```python
from build123d import *

# Parameters (mm, degrees)
F0_W     = 90
F0_H     = 55
F1_DEPTH = 35
F2_DEPTH = 7
F3_R     = 10
F4_DEPTH = 5
F6_DEPTH = 90
F7_R     = 4.99999
F8_W     = 12
F8_H     = 3
F9_DEPTH = 30.7
F10_R    = 1


# Not quite as in the source:
# - a fillet or chamfer is up to 0.001 mm smaller than in the source, because OpenCascade refuses the exact size
# - a feature names something its author has since deleted; it is built from what else it names


with BuildPart() as f1:
    # F0 (on Top) → F1 (new body)
    with BuildSketch(Plane.XY):
        Rectangle(F0_W, F0_H)
        with BuildLine():
            ThreePointArc((-40, 0), (-36.0621543344, 11.8032751438), (-25, 17.5))
            ThreePointArc((-25, 17.5), (-13.9378456656, 11.8032751438), (-10, 0))
            ThreePointArc((-10, 0), (-13.9378456656, -11.8032751438), (-25, -17.5))
            ThreePointArc((-25, -17.5), (-36.0621543344, -11.8032751438), (-40, 0))
        make_face(mode=Mode.SUBTRACT)
        with BuildLine():
            ThreePointArc((10, 0), (13.9500894873, 11.8143319509), (25.0340790777, 17.5))
            ThreePointArc((25.0340790777, 17.5), (36.0744106495, 11.7922476991), (40, 0))
            ThreePointArc((40, 0), (36.2593265414, -11.6306402206), (25.5441482581, -17.5))
            ThreePointArc((25.5441482581, -17.5), (14.1318309156, -11.9833988689), (10, 0))
        make_face(mode=Mode.SUBTRACT)
    extrude(amount=F1_DEPTH)

    # F0 (on Top) → F2 (join)
    with BuildSketch(Plane.XY):
        with BuildLine():
            ThreePointArc((-10, 0), (-13.9378456656, 11.8032751438), (-25, 17.5))
            ThreePointArc((-25, 17.5), (-36.0621543344, 11.8032751438), (-40, 0))
            ThreePointArc((-40, 0), (-36.0621543344, -11.8032751438), (-25, -17.5))
            ThreePointArc((-25, -17.5), (-13.9378456656, -11.8032751438), (-10, 0))
        make_face()
        with BuildLine():
            ThreePointArc((40, 0), (36.0744106495, 11.7922476991), (25.0340790777, 17.5))
            ThreePointArc((25.0340790777, 17.5), (13.9500894873, 11.8143319509), (10, 0))
            ThreePointArc((10, 0), (14.1318309156, -11.9833988689), (25.5441482581, -17.5))
            ThreePointArc((25.5441482581, -17.5), (36.2593265414, -11.6306402206), (40, 0))
        make_face()
    extrude(amount=F2_DEPTH)

    # F3 (on face) → F4 (cut)
    with BuildSketch(Plane.XY.offset(7)):
        with Locations((-25, 0)):
            Circle(F3_R)
        with Locations((25.2891136679, 0)):
            Circle(F3_R)
    extrude(amount=-F4_DEPTH, mode=Mode.SUBTRACT)

    # F5 (on face) → F6 (cut)
    with BuildSketch(Plane.YZ.offset(45)):
        Polygon((-27.5, 15), (27.5, 35), (-27.5, 35), align=None)
    extrude(amount=-F6_DEPTH, mode=Mode.SUBTRACT)

    # F7 (radius 5 in the source; OpenCascade refuses exactly that, so slightly less here)
    f7_edges = [f1.edges().sort_by_distance(p)[0] for p in [
        (0, 27.5, 35),
        (-45, 0, 25),
        (0, -27.5, 15),
        (45, 0, 25),
    ]]
    fillet(f7_edges, radius=F7_R)

    # F8 (on face) → F9 (cut)
    with BuildSketch(Plane.XY.offset(7)):
        with Locations((-24.9983986142, 16.138614808)):
            Rectangle(F8_W, F8_H)
        Polygon((32.0340790777, 17.5), (25.0340790777, 17.5), (18.0340790777, 17.5), (18.0340790777, 14.5), (32.0340790777, 14.5), align=None)
    extrude(amount=F9_DEPTH, mode=Mode.SUBTRACT)

    # F10
    f10_edges = [f1.edges().sort_by_distance(p)[0] for p in [
        (-24.998399, 17.638615, 31.414042),
        (-30.998399, 16.709549, 31.0762),
        (-18.998399, 16.708736, 31.075904),
        (32.034079, 16.355367, 30.947406),
        (25.034079, 17.5, 31.363636),
        (18.034079, 16.372599, 30.953672),
    ]]
    fillet(f10_edges, radius=F10_R)


solid = f1.part
```
Here's how the part is built. I have some questions about the finished solid (model axes, mm). A direction names the side the tool comes from. Give positions to 0.01 mm unless a question says otherwise; leave off trailing zeros. Write each loop counter-clockwise with the first axis right and the second up, starting at its lowest first coordinate (ties: lowest second). Pieces come first, ordered by that corner, then holes. Notation, with made-up numbers: M 45.5,-38 L 89.5,-38 A20 ccw 89.5,-22 Z; hole C 13.25,15 d8. An arc over 180 degrees is marked long. Put each result on its own line as item: value. Start each with the question number.
Item 1: Thinking about a two-plate mould opening in Y: for faces 4 (the flat face through (-1, 27.5, 14)), 5 (the cylindrical face through (43.574, 14.491, 28.669)), 6 (the flat face through (-25, 17.639, 19)), which applies, +Y half, -Y half, draft (parallel to the pull), parting line (faces both ways), or undercut?
Item 2: If we section it at A-A, the plane x = 5.5: Write out the boundary of the cut face in (y, z).
Item 3: On a 3-axis mill with a long thin cutter (end or side, diameter ignored), from which of +Z, -Z, +X, -X, +Y, -Y can I reach the whole of each face in a straight line? I mean faces 1 (the cylindrical face through (43.57, -15.02, 17.94)), 2 (the cylindrical face through (17.73, 16.45, 30.68)), 3 (the cylindrical face through (36.37, -11.495, 13.874)). Say none if no direction works.
Item 4: If we section it at C-C, the plane x = 28: Write out the boundary of the cut face in (y, z).
Item 5: Will these pins go through, and if not, where does the flat tip stop? pin 1 (6 mm diameter, centred on x = 20.5, y = -2, fed in from +Z); pin 2 (6 mm diameter, centred on y = -10, z = 19, fed in from +X); pin 3 (6 mm diameter, centred on y = -6, z = 23.5, fed in from +X); pin 4 (4 mm diameter, centred on x = -18, y = -7.5, fed in from +Z).
Item 6: If we section it at B-B, the plane z = 15: Count the separate pieces of the cut face and the enclosed holes in it, then the cut area to 3 significant figures.
Item 7: I need wall thicknesses on L1, parallel to Y at x = -25, z = 3; L2, parallel to X at y = 15.5, z = 19.5; L3, parallel to Z at x = -15.5, y = -8.5. Which ranges of each line are inside material? Lowest first, please. Write a range as from..to.
Values:
1. face 4: +Y half
1. face 5: -Y half
1. face 6: undercut
2. outline: M -27.5,0 L 27.5,0 L 27.5,27.86 A5 ccw 20.79,32.56 L -24.21,16.2 A5 ccw -27.5,11.5 Z
3. face 1: +Z, +X, -Y
3. face 2: +Z, -Y
3. face 3: +Z
4. outline: M -27.5,0 L 27.5,0 L 27.5,27.86 A5 ccw 20.79,32.56 L 18.16,31.6 A1 ccw 17.5,30.66 L 17.5,7 L 9.63,7 L 9.63,2 L -9.63,2 L -9.63,7 L -17.01,7 L -17.01,18.82 L -24.21,16.2 A5 ccw -27.5,11.5 Z
5. pin 1: z = 2
5. pin 2: x = 45
5. pin 3: x = 44.25
5. pin 4: z = 7
6. separate pieces: 1
6. enclosed holes: 2
6. area: 3,130 mm²
7. L1: -27.5..-10, 10..27.5
7. L2: -45..-31.53, -18.47..18.03, 32.03..45
7. L3: 0..7
